Autodesk Inventor part; units mm, degrees
ref_plane "YZ Plane" through (0, 0, 0) normal (1, 0, 0) x (0, 1, 0)
ref_plane "XZ Plane" through (0, 0, 0) normal (0, 1, 0) x (-1, 0, 0)
ref_plane "XY Plane" through (0, 0, 0) normal (0, 0, 1) x (1, 0, 0)
sketch "Sketch1" plane through (0, 0, 0) normal (0, 1, 0) x (-1, 0, 0)
  line L0 (88.9, 254) -> (-88.9, 254)
  line L1 (-88.9, -254) -> (88.9, -254)
  line L2 (0, -266.7) -> (0, 266.7)
  line L3 (-444.5, 0) -> (444.5, 0)
  line L4 (88.9, -88.9) -> (317.5, -88.9)
  line L5 (317.5, -88.9) -> (317.5, 88.9)
  line L6 (317.5, 88.9) -> (88.9, 88.9)
  line L7 (-88.9, 88.9) -> (-317.5, 88.9)
  line L8 (-317.5, 88.9) -> (-317.5, -88.9)
  line L9 (-317.5, -88.9) -> (-88.9, -88.9)
  line L10 (88.9, -254) -> (88.9, -88.9)
  line L11 (88.9, 88.9) -> (88.9, 254)
  line L12 (-88.9, 254) -> (-88.9, 88.9)
  line L13 (-88.9, -88.9) -> (-88.9, -254)
  line L14 (88.9, -88.9) -> (88.9, 88.9)
  line L15 (-88.9, -88.9) -> (-88.9, 88.9)
  line L16 (88.9, -88.9) -> (-88.9, -88.9)
  line L17 (-88.9, 88.9) -> (88.9, 88.9)
  point P0 (0, 0)
  dimension "d1" = 177.8
  dimension "d5" = 177.8
  dimension "d6" = 635
  dimension "d7" = 508
extrude "Extrusion1" add sketch "Sketch1" along normal blind 6.35
equation "\"d1\" = Height"
equation "\"d5\" = Width"
equation "\"d6\" = HLength"
equation "\"d7\" = WLength"
equation "\"HLength\" = 635"
equation "\"Height\" = 177.8"
equation "\"Width\" = 177.8"
equation "\"WLength\" = 508"
properties part number "Electronics Board"
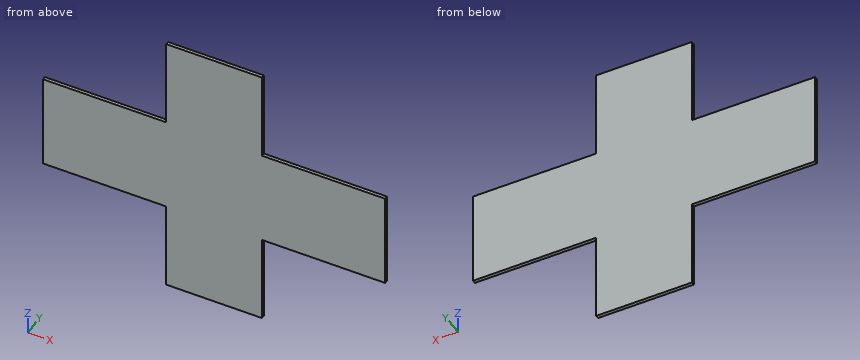
The model under review builds one solid part; all positions refer to its coordinate system, in mm. Coordinates: 2 decimals unless noted, no trailing zeros. Write each loop counter-clockwise with the first axis right and the second up, starting at its lowest first coordinate (ties: lowest second). Pieces come first, ordered by that corner, then holes. Notation, with made-up numbers: (20, 49.25) - (77, 49.25) arc R14 cw to (77, 71.25) - close; hole circle Ø1 at (6, 19.5). An arc over 180 degrees is marked (long way). Answer as a JSON object with one key per item and string values. Group by question number.
1. Clearance check with flat-ended pins moving along their axes: pin 1 Ø3 at (y, z) = (4, 165) entering from +X; pin 2 Ø2 at (x, y) = (164, 2) entering from +Z; pin 3 Ø1.5 at (x, y) = (-91.5, 4) entering from -Z. State where each tip first meets the part, or that it passes through.
2. Add section B-B (x = -125). Give the boundary of the cut face in (y, z), plus the area to 3 significant figures.
3. Add section C-C (z = -127). Give the boundary of the cut face in (x, y).
4. To check wall thickness, follow probe 1 along X at (y, z) = (4.5, -96.5). State the ranges of the line that lie inside material, in increasing order.
5. Add section A-A (y = 2.5). Give the boundary of the cut face in (x, z), plus the area to 3 significant figures.
Findings:
{
 "1": {"pin 1": "x = 88.9", "pin 2": "z = 88.9", "pin 3": "z = -88.9"},
 "2": {"outline": "(0, -88.9) - (6.35, -88.9) - (6.35, 88.9) - (0, 88.9) - close", "area": "1,130 mm²"},
 "3": {"outline": "(-88.9, 0) - (88.9, 0) - (88.9, 6.35) - (-88.9, 6.35) - close"},
 "4": {"probe 1": "-88.9 to 88.9"},
 "5": {"outline": "(-317.5, -88.9) - (-88.9, -88.9) - (-88.9, -254) - (88.9, -254) - (88.9, -88.9) - (317.5, -88.9) - (317.5, 88.9) - (88.9, 88.9) - (88.9, 254) - (-88.9, 254) - (-88.9, 88.9) - (-317.5, 88.9) - close", "area": "172,000 mm²"}
}
